Can you work these out from the model? Positions are in its coordinate system, mm. A direction names the side the tool comes from. Coordinates: 2 decimals unless noted, no trailing zeros. Order: outer loops, then holes, each group sorted by start corner. A loop starts at its lowest first (then second) coordinate and runs counter-clockwise, first axis right, second up. Notation, with made-up numbers: M 7.5,41.25 L 22.5,41.25 A22 cw 22.5,61.25 Z; hole C 34,35.5 d10. An arc over 180 degrees is marked long. Answer as a JSON object with one key per item and string values.
from build123d import *

# Parameters (mm, degrees)
F0_W         = 34.925
F0_H         = 12.7
F1_DEPTH     = 9.7155
F3_R         = 1.5875
F4_DEPTH     = 25.4
F5_SIZE      = 0.79375
F6_T1_DEPTH  = 34.2562991577
F7_SIZE      = 0.79375
F11_R        = 7.493
F12_DEPTH    = 50.8
F13_T1_DEPTH = 15.1455192093
F13_T3_DEPTH = 15.1455192093


# Not quite as in the source:
# - a fillet or chamfer that OpenCascade refuses, or shapes differently, is made with other operations: its cross-section is extruded or revolved along the edge and cut away or added


with BuildPart() as f1:
    # F0 (on Top) → F1 (new body)
    with BuildSketch(Plane.XY):
        with Locations((-17.4625, 6.35)):
            Rectangle(F0_W, F0_H)
        with Locations((17.4625, 6.35)):
            Rectangle(F0_W, F0_H)
    extrude(amount=F1_DEPTH)

    # F3 (on face) → F4 (cut)
    with BuildSketch(Plane(origin=(0, 12.7, 0), x_dir=(-1, 0, 0), z_dir=(0, 1, 0))):
        with Locations((16.51, 4.71678)):
            Circle(F3_R)
        with Locations((-16.51, 4.71678)):
            Circle(F3_R)
    extrude(amount=-F4_DEPTH, mode=Mode.SUBTRACT)

    # F5
    f5_edges = [f1.edges().sort_by_distance(p)[0] for p in [
        (-34.925, 6.35, 9.7155),
        (34.925, 6.35, 9.7155),
        (0, 12.7, 9.7155),
        (0, 12.7, 0),
        (-34.925, 6.35, 0),
        (34.925, 6.35, 0),
    ]]
    chamfer(f5_edges, length=F5_SIZE)

    # F6: chamfer of 5.08 on 2 edges, made by hand

    # F6_s2 → F6_t1 (cut)
    with BuildSketch(Plane.XY.offset(-12.2703995789)):
        Polygon((34.925, 7.62), (29.845, 12.7), (34.925, 12.7), align=None)
        Polygon((-34.925, 7.62), (-29.845, 12.7), (-34.925, 12.7), align=None)
    extrude(amount=F6_T1_DEPTH, mode=Mode.SUBTRACT)

    # F7
    f7_edges = [f1.edges().sort_by_distance(p)[0] for p in [
        (32.385, 10.16, 0),
        (32.385, 10.16, 9.7155),
        (-32.385, 10.16, 9.7155),
        (-32.385, 10.16, 0),
    ]]
    chamfer(f7_edges, length=F7_SIZE)

    # F11 (on face) → F12 (cut)
    with BuildSketch(Plane(origin=(-8.3875461679, 0, -14.5276561136), x_dir=(0.8660254038, 0, -0.5), z_dir=(0.5, 0, 0.8660254038))):
        with Locations((-2.3805295629, 0)):
            Circle(F11_R)
    extrude(amount=F12_DEPTH, mode=Mode.SUBTRACT)

    # F13: chamfer of 0.8001 on 2 edges, made by hand

    # F13_s2 → F13_t1 (cut)
    with BuildSketch(Plane(origin=(3.740760597, 0, 6.4791874129), x_dir=(0, 1, 0), z_dir=(-0.5, 0, -0.8660254038))):
        with BuildLine():
            Line((0, -10.6349433883), (0.7229081164, -9.8385757451))
            ThreePointArc((0.7229081164, -9.8385757451), (0.3732081581, -9.8642294948), (0, -9.8735295629))
            Line((0, -9.8735295629), (0, -10.6349433883))
        make_face()
    extrude(amount=F13_T1_DEPTH, mode=Mode.SUBTRACT)

    # F13_s4 → F13_t3 (cut)
    with BuildSketch(Plane(origin=(0.4940865594, 0, 0.8557830242), x_dir=(0, 1, 0), z_dir=(0.5, 0, 0.8660254038))):
        with BuildLine():
            Line((0, -5.8738842624), (0.7229081164, -5.0775166192))
            ThreePointArc((0.7229081164, -5.0775166192), (0.3732081581, -5.103170369), (0, -5.1124704371))
            Line((0, -5.1124704371), (0, -5.8738842624))
        make_face()
    extrude(amount=F13_T3_DEPTH, mode=Mode.SUBTRACT)


solid = f1.part
Item 1: If we mould it in two halves opening along X, with no side actions, what happens to faces 1 (the cylindrical face through (0.12, 7.49, 4.66)), 2 (the flat face through (-34.925, 4, 5)), 3 (the flat face through (32.421, 10.124, 4.801))? For each: pulls with the +X half, pulls with the -X half, needs draft (parallel to the pull), parting line crosses it, or undercut.
Answers follow:
{"face 1": "undercut", "face 2": "pulls with the -X half", "face 3": "pulls with the +X half"}
Item 2: Which directions (+Z, -Z, +X, -X, +Y, -Y) give clear straight access to the entire face, cutting with the end or side of a thin tool? Please do faces 4 (the flat face through (9.091, 0.356, 4.784)), 5 (the flat face through (-8.98, 0.356, 4.931)), 6 (the flat face through (-32.065, 9.911, 9.324)).
Answers follow:
{"face 4": "+Z, -Y", "face 5": "-Z, -Y", "face 6": "+Z, -X, +Y"}
Item 3: I'm going to push flat-ended pins straight in: pin 1 (1 mm diameter, centred on x = 2.5, z = 6.5, fed in from -Y); pin 2 (1 mm diameter, centred on y = 8.5, z = 6.5, fed in from +X) (3 decimals). Where does each tip first touch, or does it pass through?
Answers follow:
{"pin 1": "stops at y = 7.27", "pin 2": "stops at x = 34.545"}
Item 4: Please list where these lines run through material, in increasing order: line 1 (Z direction, x = 16.51, y = 7.75); line 2 (X direction, y = 3.5, z = 4.75) (3 decimals); line 3 (X direction, y = 7.75, z = 6) (3 decimals).
Answers follow:
{"line 1": "z = 0 to 3.13, 6.3 to 9.72", "line 2": "x = -34.925 to -18.097, -14.923 to -7.657, 7.644 to 14.923, 18.097 to 34.925", "line 3": "x = -34.795 to -17.445, -15.575 to 15.575, 17.445 to 34.795"}
Item 5: I want a section at A-A, the plane x = 16.51. Write out the boundary of the cut face in (y, z), plus the area to 3 significant figures.
Answers follow:
{"outline": "M 0,0 L 11.91,0 L 12.7,0.79 L 12.7,3.13 L 0,3.13 Z; M 0,6.3 L 12.7,6.3 L 12.7,8.92 L 11.91,9.72 L 0,9.72 Z", "area": "82.4 mm^2"}
Item 6: I want a section at B-B, the plane y = 9.75. Write out the boundary of the cut face in (x, z) (1 decimal).
Answers follow:
{"outline": "M -32.8,0.8 L -31.7,0 L 31.7,0 L 32.8,0.8 L 32.8,8.9 L 31.7,9.7 L -31.7,9.7 L -32.8,8.9 Z; hole C -16.5,4.7 d3.2; hole C 16.5,4.7 d3.2"}
